Autodesk Inventor part; units mm, degrees
ref_plane "YZ Plane" through (0, 0, 0) normal (1, 0, 0) x (0, 1, 0)
ref_plane "XZ Plane" through (0, 0, 0) normal (0, 1, 0) x (-1, 0, 0)
ref_plane "XY Plane" through (0, 0, 0) normal (0, 0, 1) x (1, 0, 0)
sketch "Sketch1" plane through (0, 0, 0) normal (0, 1, 0) x (-1, 0, 0)
  line L0 (0, 0) -> (-20, 0)
  line L1 (-20, 0) -> (-20, -60)
  line L2 (-20, -60) -> (0, -60)
  line L3 (0, -60) -> (0, 0)
  dimension "d0" = 20
  dimension "d1" = 60
extrude "Extrusion1" add sketch "Sketch1" along normal blind 5
sketch "Sketch2" plane through (0, 5, 0) normal (0, 1, 0) x (1, 0, 0)
  line L0 (0, 0) -> (20, 0)
  line L1 (10, 0) -> (10, 9)
  line L2 (10, 0) -> (19, 0) construction
  circle A0 centre (10, 9) radius 5
  line L3 (20, 60) -> (0, 60)
  line L4 (0, 0) -> (0, 60)
  line L5 (0, 60) -> (0, 0)
  line L6 (0, 30) -> (2.0385, 30)
  circle A1 centre (10, 51) radius 5
  dimension "d5" = 9
  dimension "d6" = 90
  dimension "d7" = 10
extrude "Extrusion2" cut sketch "Sketch2" against normal blind 23
properties part number "BaseBancada"
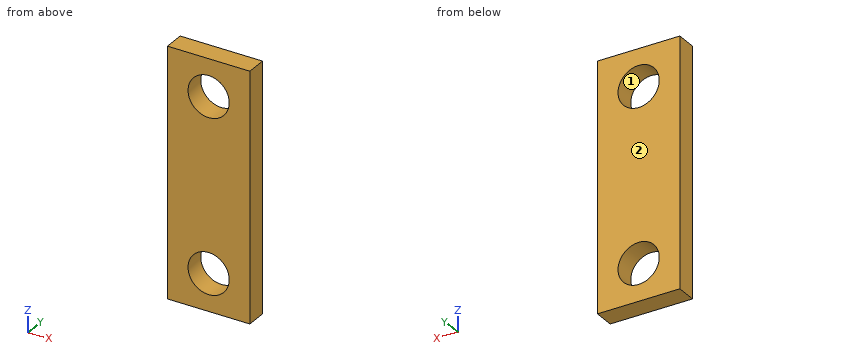
Can you work these out from the model? Positions are in its coordinate system, mm. Face numbers are marked on the shaded views. Give positions to 0.01 mm unless a question says otherwise; leave off trailing zeros. Loops run counter-clockwise (first coordinate to the right, second up) from the corner with the lowest first, then second, coordinate; pieces in that order, holes last. Notation, with made-up numbers: (37.25, -13) - (65.25, -13) arc R16 cw to (65.25, 17) - close; hole circle Ø3 at (79, 48.25). An arc over 180 degrees is marked (long way). One line per item, written item: value.
(1) If we mould it in two halves opening along X, with no side actions, what happens to the marked faces 1 and 2? For each: released by +X, released by -X, zero draft, split by the parting line, or undercut.
Verdict:
face 1: undercut
face 2: zero draft
(2) If we section it at C-C, the plane y = 1.55: List the corners of the cut face in (x, z) for me.
Verdict:
outline: (0, -60) - (20, -60) - (20, 0) - (0, 0) - close; hole circle Ø10 at (10, -51); hole circle Ø10 at (10, -9)
(3) If we section it at D-D, the plane x = 5.75: List the corners of the cut face in (y, z) for me.
Verdict:
outline: (0, -60) - (5, -60) - (5, -53.63) - (0, -53.63) - close; (0, -48.37) - (5, -48.37) - (5, -11.63) - (0, -11.63) - close; (0, -6.37) - (5, -6.37) - (5, 0) - (0, 0) - close
(4) If we section it at B-B, the plane z = -48: List the corners of the cut face in (x, y) for me, plus the area to 3 significant figures.
Verdict:
outline: (0, 0) - (6, 0) - (6, 5) - (0, 5) - close; (14, 0) - (20, 0) - (20, 5) - (14, 5) - close
area: 60.0 mm^2
(5) I need wall thicknesses on line 1 along Z through (x, y) = (10, 2.45); line 2 along X through (y, z) = (4, -9); line 3 along Z through (x, y) = (9.25, 4.4). Which ranges of each line are inside material? Lowest first, please.
Verdict:
line 1: -60 to -56, -46 to -14, -4 to 0
line 2: 0 to 5, 15 to 20
line 3: -60 to -55.94, -46.06 to -13.94, -4.06 to 0
(6) If we section it at A-A, the plane x = 10: List the corners of the cut face in (y, z) for me.
Verdict:
outline: (0, -60) - (5, -60) - (5, -56) - (0, -56) - close; (0, -46) - (5, -46) - (5, -14) - (0, -14) - close; (0, -4) - (5, -4) - (5, 0) - (0, 0) - close
